Print and shaded views of the part. All mm, measured from the part's lowest x, y and z. Give positions to 0.01 mm unless a question says otherwise; leave off trailing zeros. Write each loop counter-clockwise with the first axis right and the second up, starting at its lowest first coordinate (ties: lowest second). Pieces come first, ordered by that corner, then holes. Notation, with made-up numbers: (12, -10) -> (39, -10) arc R14 cw to (39, -5) -> close; hole circle Ø4 at (43, 49.5). An arc over 180 degrees is marked (long way). Put each result on its own line as item: value.
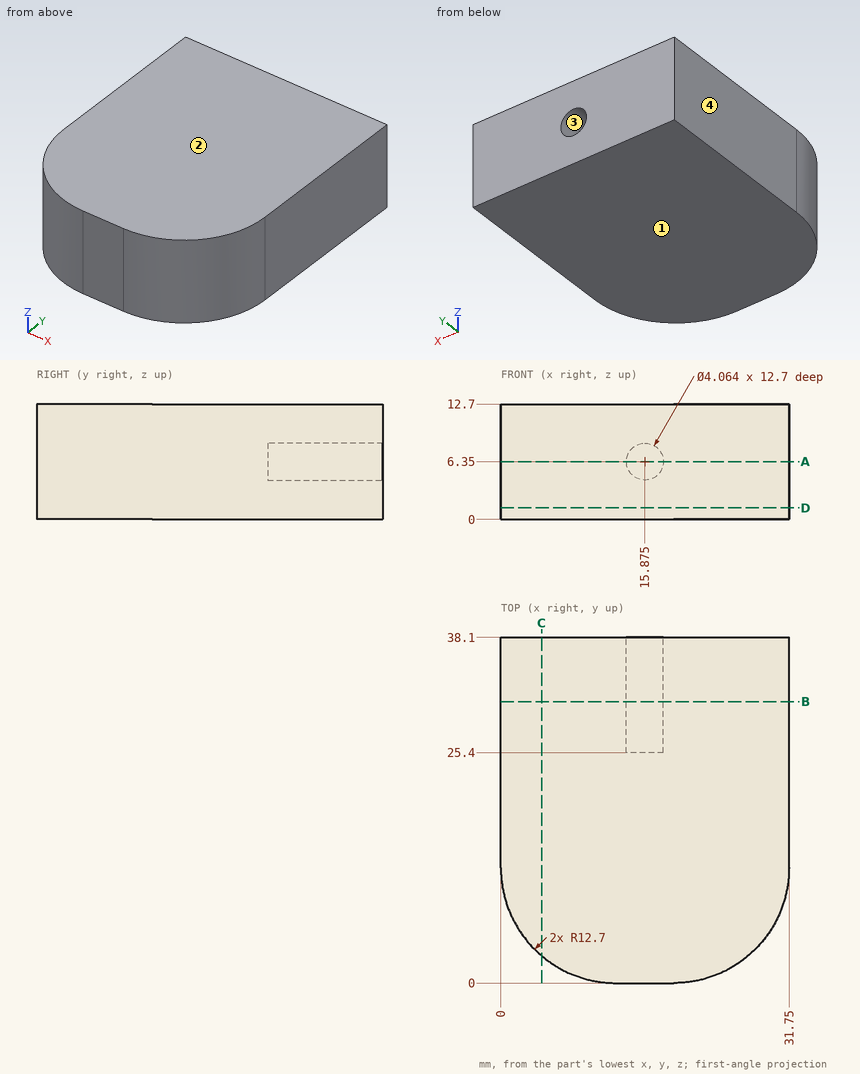
1) Wall check: L1, parallel to X at y = 32, z = 6.35; L2, parallel to X at y = 33.5, z = 8; L3, parallel to Y at x = 11, z = 11.5. Give the ranges that are in metal, low to high.
Filled sheet:
L1: 0 to 13.84, 17.91 to 31.75
L2: 0 to 14.69, 17.06 to 31.75
L3: 0.11 to 38.1
2) Slice it at A-A (z = 6.35). Write the cut outline in (x, y), plus the area to 3 significant figures.
Filled sheet:
outline: (0, 12.7) arc R12.7 ccw to (12.7, 0) -> (19.05, 0) arc R12.7 ccw to (31.75, 12.7) -> (31.75, 38.1) -> (17.91, 38.1) -> (17.91, 25.4) -> (13.84, 25.4) -> (13.84, 38.1) -> (0, 38.1) -> close
area: 1,090 mm2
3) Pin check, flat tips, straight feed: pin 1 (1.2 mm diameter, centred on x = 15.5, z = 6, fed in from +Y); pin 2 (6 mm diameter, centred on x = 26, z = 4.5, fed in from -Y); pin 3 (4 mm diameter, centred on x = 6.5, z = 8, fed in from -Y). Stop position of each tip, or through.
Filled sheet:
pin 1: y = 25.4
pin 2: y = 0.63
pin 3: y = 0.71
4) Slice it at D-D (z = 1.25). Write the cut outline in (x, y), plus the area to 3 significant figures.
Filled sheet:
outline: (0, 12.7) arc R12.7 ccw to (12.7, 0) -> (19.05, 0) arc R12.7 ccw to (31.75, 12.7) -> (31.75, 38.1) -> (0, 38.1) -> close
area: 1,140 mm2
5) Pull direction Z, two halves, no side cores. Call the marked faces 1, 2, 3 and 4: released by +Z, released by -Z, zero draft, split by the parting line, or undercut.
Filled sheet:
face 1: released by -Z
face 2: released by +Z
face 3: undercut
face 4: zero draft
6) Slice it at B-B (y = 31). Write the cut outline in (x, z) (3 decimals).
Filled sheet:
outline: (0, 0) -> (31.75, 0) -> (31.75, 12.7) -> (0, 12.7) -> close; hole circle Ø4.064 at (15.875, 6.35)
7) Slice it at C-C (x = 4.5). Write the cut outline in (y, z), plus the area to 3 significant figures.
Filled sheet:
outline: (3, 0) -> (38.1, 0) -> (38.1, 12.7) -> (3, 12.7) -> close
area: 446 mm2
